Part model, mm, in its own coordinate system. A direction names the side the tool comes from. Round coordinates to 2 decimals unless told otherwise and drop trailing zeros. Write each loop counter-clockwise with the first axis right and the second up, starting at its lowest first coordinate (ties: lowest second). Pieces come first, ordered by that corner, then holes. Notation, with made-up numbers: M 81.5,-16 L 91.5,-16 A31 ccw 91.5,20 Z; hole C 52.5,-18 d9. An arc over 180 degrees is marked long. One line per question, with ' | ' between items. Start each with the question number.
1) Drop flat-ended pins along their axis: pin 1 Ø10 at (x, z) = (-212.5, 20.5) entering from -Y; pin 2 Ø4.5 at (x, y) = (-230.54, 15.65) entering from +Z (3 decimals); pin 3 Ø6.5 at (x, z) = (-217.84, 8.26) entering from -Y. Give the stop position or say it passes through.
2) Saw through at B-B (x = -218.5). List the corners of the cut face in (y, z) (1 decimal), plus the area to 3 significant figures.
3) Saw through at C-C (z = 9.75). List the corners of the cut face in (x, y).
4) Saw through at A-A (y = 14.5). List the corners of the cut face in (x, z) (3 decimals).
5) Saw through at D-D (x = -233.5). List the corners of the cut face in (y, z) (1 decimal), plus the area to 3 significant figures.
6) Tool access for faces 4 (the face through (-209.586, 28, 7)), 5 (the face through (-211.491, 28, 9)): list every direction of +Z, -Z, +X, -X, +Y, -Y with a clear straight run to the whole face (end or side of a thin tool).
7) Mould opens along Z. For faces 1 (the face through (-219.82, 35.63, 8.34)), 2 (the face through (-224, 22, 1.905)), 3 (the face through (-236.891, 28, 9)) say: pulls with the +Z half, pulls with the -Z half, needs draft (parallel to the pull), parting line crosses it, or undercut.
8) Wall check: probe 1 along X at (y, z) = (28.75, 10.25); probe 2 along Y at (x, z) = (-229.25, 12.5); probe 3 along Z at (x, y) = (-228.75, 10.75) (3 decimals). Give the ranges that are in metal, low to high. Write a range as [from, to].
```python
from build123d import *

# Parameters (mm, degrees)
F0_W     = 29.21
F0_H     = 29.21
F1_DEPTH = 27.305
F4_DEPTH = 25.4
F5_DEPTH = 29.21
F6_R     = 1.9812
F8_DEPTH = 25.4
F7_R     = 1.9812
F9_DEPTH = 25.4


with BuildPart() as f1:
    # F0 (on Top) → F1 (new body)
    with BuildSketch(Plane.XY):
        with Locations((-224.190711, 21.995599)):
            Rectangle(F0_W, F0_H)
    extrude(amount=F1_DEPTH)

    # F2 (on face) → F4 (cut)
    with BuildSketch(Plane.XY.offset(27.305)):
        Polygon((-236.890711, 34.695599), (-236.890711, 7.390599), (-211.490711, 7.390599), (-211.490711, 34.695599), (-224.190711, 34.695599), align=None)
    extrude(amount=-F4_DEPTH, mode=Mode.SUBTRACT)

    # F3 (on face) → F5 (cut)
    with BuildSketch(Plane(origin=(-238.795711, 0, 0), x_dir=(0, -1, 0), z_dir=(-1, 0, 0))):
        Polygon((-7.390599, 27.305), (-36.600599, 27.305), (-7.390599, 0), align=None)
    extrude(amount=-F5_DEPTH, mode=Mode.SUBTRACT)

    # F6 (on face) → F8 (cut)
    with BuildSketch(Plane.XY.offset(1.905)):
        with Locations((-230.540711, 28.345599)):
            Circle(F6_R)
        with Locations((-217.840711, 28.345599)):
            Circle(F6_R)
        with Locations((-217.840711, 15.645599)):
            Circle(F6_R)
        with Locations((-230.540711, 15.645599)):
            Circle(F6_R)
    extrude(amount=-F8_DEPTH, mode=Mode.SUBTRACT)

    # F7 (on face) → F9 (cut)
    with BuildSketch(Plane.XZ.offset(-34.695599)):
        with Locations((-230.540711, 8.255)):
            Circle(F7_R)
        with Locations((-230.540711, 20.955)):
            Circle(F7_R)
        with Locations((-217.840711, 20.955)):
            Circle(F7_R)
        with Locations((-217.840711, 8.255)):
            Circle(F7_R)
    extrude(amount=-F9_DEPTH, mode=Mode.SUBTRACT)


solid = f1.part
```
Answer key:
1) pin 1: stops at y = 24.08 | pin 2: stops at z = 1.905 | pin 3: stops at y = 34.7
2) outline: M 7.4,0 L 13.8,0 L 13.8,1.9 L 9.4,1.9 Z; M 17.5,0 L 26.5,0 L 26.5,1.9 L 17.5,1.9 Z; M 30.2,0 L 36.6,0 L 36.6,6.4 L 34.7,6.4 L 34.7,1.9 L 30.2,1.9 Z; M 34.7,10.1 L 36.6,10.1 L 36.6,19.1 L 34.7,19.1 Z; M 34.7,22.8 L 36.6,22.8 L 36.6,27.3 L 34.7,25.5 Z | area: 71.9 mm2
3) outline: M -238.8,17.82 L -236.89,17.82 L -236.89,34.7 L -231.84,34.7 L -231.84,36.6 L -238.8,36.6 Z; M -229.24,34.7 L -219.14,34.7 L -219.14,36.6 L -229.24,36.6 Z; M -216.54,34.7 L -211.49,34.7 L -211.49,17.82 L -209.59,17.82 L -209.59,36.6 L -216.54,36.6 Z
4) outline: M -238.796,0 L -232.157,0 L -232.157,1.905 L -236.891,1.905 L -236.891,6.646 L -238.796,6.646 Z; M -228.924,0 L -219.457,0 L -219.457,1.905 L -228.924,1.905 Z; M -216.224,0 L -209.586,0 L -209.586,6.646 L -211.491,6.646 L -211.491,1.905 L -216.224,1.905 Z
5) outline: M 7.4,0 L 36.6,0 L 36.6,27.3 L 34.7,25.5 L 34.7,1.9 L 9.4,1.9 Z | area: 100 mm2
6) face 4: +Z, -Z, +X, +Y, -Y | face 5: +Z, -Y
7) face 1: undercut | face 2: pulls with the +Z half | face 3: needs draft
8) probe 1: x = [-238.8, -236.89], [-211.49, -209.59] | probe 2: y = [34.7, 36.6] | probe 3: z = [0, 1.905]
